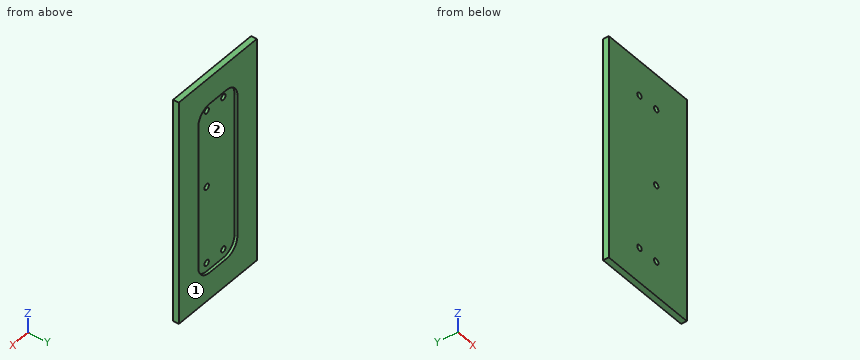
```python
from build123d import *

# Parameters (mm, degrees)
F0_W     = 35
F0_H     = 80
F1_DEPTH = 2
F2_W     = 17.5
F2_H     = 61
F3_DEPTH = 1
F4_R     = 1
F5_DEPTH = 25
F6_R     = 5


with BuildPart() as f1:
    # F0 (on Front) → F1 (new body)
    with BuildSketch(Plane.XZ):
        Rectangle(F0_W, F0_H)
    extrude(amount=F1_DEPTH)

    # F2 (on face) → F3 (cut)
    with BuildSketch(Plane(origin=(0, 0, 0), x_dir=(-1, 0, 0), z_dir=(0, 1, 0))):
        Rectangle(F2_W, F2_H)
    extrude(amount=-F3_DEPTH, mode=Mode.SUBTRACT)

    # F4 (on face) → F5 (cut)
    with BuildSketch(Plane(origin=(0, -1, 0), x_dir=(-1, 0, 0), z_dir=(0, 1, 0))):
        with Locations((-3.75, 27.5)):
            Circle(F4_R)
        with Locations((-3.75, 0)):
            Circle(F4_R)
        with Locations((-3.75, -27.5)):
            Circle(F4_R)
        with Locations((3.75, 27.5)):
            Circle(F4_R)
        with Locations((3.75, -27.5)):
            Circle(F4_R)
    extrude(amount=-F5_DEPTH, mode=Mode.SUBTRACT)

    # F6
    f6_edges = [f1.edges().sort_by_distance(p)[0] for p in [
        (-8.75, -0.5, 30.5),
        (8.75, -0.5, 30.5),
        (-8.75, -0.5, -30.5),
        (8.75, -0.5, -30.5),
    ]]
    fillet(f6_edges, radius=F6_R)


solid = f1.part
```
Model file for the job. Use its own axes, mm. Face numbers are marked on the shaded views. Round coordinates to 2 decimals unless told otherwise and drop trailing zeros. Write each loop counter-clockwise with the first axis right and the second up, starting at its lowest first coordinate (ties: lowest second). Pieces come first, ordered by that corner, then holes. Notation, with made-up numbers: M -15,23 L 35,23 A18 ccw 35,49 Z; hole C 87,83 d6. An arc over 180 degrees is marked long. Put each result on its own line as item: value.
Item 1: Cut at B-B (y = -0.4). List the corners of the cut face in (x, z), and give its area (3 significant figures).
Responses:
outline: M -17.5,-40 L 17.5,-40 L 17.5,40 L -17.5,40 Z; hole M -8.75,-25.5 A5 ccw -3.75,-30.5 L 3.75,-30.5 A5 ccw 8.75,-25.5 L 8.75,25.5 A5 ccw 3.75,30.5 L -3.75,30.5 A5 ccw -8.75,25.5 Z
area: 1,750 mm²
Item 2: Cut at A-A (z = 0). List the corners of the cut face in (x, y).
Responses:
outline: M -17.5,-2 L 2.75,-2 L 2.75,-1 L -8.75,-1 L -8.75,0 L -17.5,0 Z; M 4.75,-2 L 17.5,-2 L 17.5,0 L 8.75,0 L 8.75,-1 L 4.75,-1 Z
Item 3: Flat gauge pin, fed straight in: P1, Ø1.6, axis at x = 3.75, z = -27.5, coming from the +Y side. Where does the tip first touch, or does it go through?
Responses:
P1: through
Item 4: Probe L1, parallel to Z at x = -3.75, y = -1.6; L2, parallel to Z at x = 3.75, y = -1.65; L3, parallel to Z at x = 0, y = -0.05. List the from-to ranges inside material, lowest first. Write a range as from..to.
Responses:
L1: -40..-28.5, -26.5..26.5, 28.5..40
L2: -40..-28.5, -26.5..-1, 1..26.5, 28.5..40
L3: -40..-30.5, 30.5..40
Item 5: Mould opens along Z. For the marked faces 1 and 2 say: +Z half, -Z half, draft (parallel to the pull), parting line (faces both ways), or undercut.
Responses:
face 1: draft
face 2: undercut
Item 6: Cut at D-D (x = -6.5). List the corners of the cut face in (y, z).
Responses:
outline: M -2,-40 L 0,-40 L 0,-29.68 L -1,-29.68 L -1,29.68 L 0,29.68 L 0,40 L -2,40 Z
Item 7: Cut at C-C (z = -18). List the corners of the cut face in (x, y).
Responses:
outline: M -17.5,-2 L 17.5,-2 L 17.5,0 L 8.75,0 L 8.75,-1 L -8.75,-1 L -8.75,0 L -17.5,0 Z
